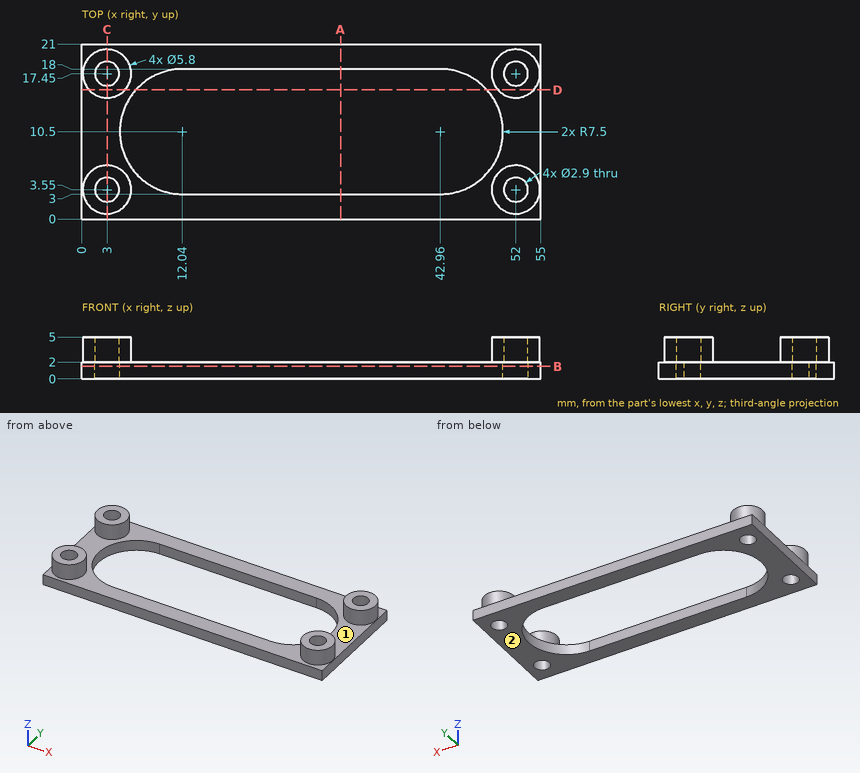
Check sheet for the drawn part. Datum: minimum x, y, z corner. Units: mm. A direction names the side the tool comes from. Give positions to 0.01 mm unless a question says otherwise; leave off trailing zeros. Order: outer loops, then holes, each group sorted by start corner. A loop starts at its lowest first (then second) coordinate and runs counter-clockwise, first axis right, second up.
1. Sectioned sample at D-D (y = 15.5). Record the boundary of the cut face in (x, z).
Completed:
outline: (0, 0) - (6.45, 0) - (6.45, 2) - (5.15, 2) - (5.15, 5) - (0.85, 5) - (0.85, 2) - (0, 2) - close; (48.55, 0) - (55, 0) - (55, 2) - (54.15, 2) - (54.15, 5) - (49.85, 5) - (49.85, 2) - (48.55, 2) - close
2. Sectioned sample at C-C (x = 3). Record the boundary of the cut face in (y, z), then the cut area to 3 significant figures.
Completed:
outline: (0, 0) - (2.1, 0) - (2.1, 5) - (0.65, 5) - (0.65, 2) - (0, 2) - close; (5, 0) - (16, 0) - (16, 5) - (14.55, 5) - (14.55, 2) - (6.45, 2) - (6.45, 5) - (5, 5) - close; (18.9, 0) - (21, 0) - (21, 2) - (20.35, 2) - (20.35, 5) - (18.9, 5) - close
area: 47.8 mm2
3. Sectioned sample at B-B (z = 1.5). Record the boundary of the cut face in (x, y).
Completed:
outline: (0, 0) - (55, 0) - (55, 21) - (0, 21) - close; hole circle Ø2.9 at (3, 3.55); hole circle Ø2.9 at (3, 17.45); hole (12.04, 3) - (42.96, 3) arc R7.5 ccw to (42.96, 18) - (12.04, 18) arc R7.5 ccw to start; hole circle Ø2.9 at (52, 3.55); hole circle Ø2.9 at (52, 17.45)
4. Access from +Z, -Z, +X, -X, +Y, -Y to the whole of each face (thin tool, end or side, straight path). Record for the marked faces 1 and 2.
Completed:
face 1: +Z
face 2: -Z, +X, -X, +Y, -Y
5. Scan lines: line 1 (Y direction, x = 3, z = 1.55); line 2 (Y direction, x = 52, z = 3.4); line 3 (Y direction, x = 38.5, z = 0.3). Record each from-to range of solid material in increasing order.
Completed:
line 1: y = 0 to 2.1, 5 to 16, 18.9 to 21
line 2: y = 0.65 to 2.1, 5 to 6.45, 14.55 to 16, 18.9 to 20.35
line 3: y = 0 to 3, 18 to 21
6. Depth check by flat-ended pin: pin 1 (1.7 mm diameter, centred on x = 3, y = 17.45, fed in from -Z); pin 2 (1 mm diameter, centred on y = 6.5, z = 3.5, fed in from -X). Enter the tip coordinate at first touch or a pass-through.
Completed:
pin 1: passes through
pin 2: stops at x = 1.45
7. Sectioned sample at A-A (x = 31). Record the boundary of the cut face in (y, z).
Completed:
outline: (0, 0) - (3, 0) - (3, 2) - (0, 2) - close; (18, 0) - (21, 0) - (21, 2) - (18, 2) - close
